```python
from build123d import *

# Parameters (mm, degrees)
F0_W     = 25
F0_H     = 300
F0_R     = 7.5
F0_R_2   = 4.25
F1_DEPTH = 50


with BuildPart() as f1:
    # F0 (on Top) → F1 (new body, symmetric)
    with BuildSketch(Plane.XY):
        Rectangle(F0_W, F0_H)
        with Locations((0, -115)):
            Circle(F0_R, mode=Mode.SUBTRACT)
        Circle(F0_R_2, mode=Mode.SUBTRACT)
        with Locations((0, 115)):
            Circle(F0_R, mode=Mode.SUBTRACT)
    extrude(amount=F1_DEPTH, both=True)


solid = f1.part
```
Read the model definition and answer for the solid it produces. Units are mm, in the model's axes. Give positions to 0.01 mm unless a question says otherwise; leave off trailing zeros. Order: outer loops, then holes, each group sorted by start corner. A loop starts at its lowest first (then second) coordinate and runs counter-clockwise, first axis right, second up.
(1) Find section D-D (y = 0). Give the vertices of the cut face in (x, z), plus the area to 3 significant figures.
(2) Find section B-B (x = 0). Give the vertices of the cut face in (y, z).
(3) Straight lines are drawn through the part: L1, parallel to Y at x = 0, z = 7; L2, parallel to Y at x = -3, z = -19.5; L3, parallel to Y at x = -6, z = 9. For each, find the intervals that lie inside material, in ascending order.
(4) For a pull along Y with two mould halves and no side action, classify faces 1 (the flat face through (0, -150, 1)), 2 (the flat face through (-6, 2, 50)), 3 (the cylindrical face through (-1.63, -122.32, -0.7)) as released by +Y, released by -Y, zero draft, split by the parting line, or undercut.
(5) Find section A-A (y = -115). Give the vertices of the cut face in (x, z).
(6) Find section C-C (z = -38.5). Give the vertices of the cut face in (x, y), plus the area to 3 significant figures.
Result sheet:
1. outline: (-12.5, -50) - (-4.25, -50) - (-4.25, 50) - (-12.5, 50) - close; (4.25, -50) - (12.5, -50) - (12.5, 50) - (4.25, 50) - close
1. area: 1,650 mm2
2. outline: (-150, -50) - (-122.5, -50) - (-122.5, 50) - (-150, 50) - close; (-107.5, -50) - (-4.25, -50) - (-4.25, 50) - (-107.5, 50) - close; (4.25, -50) - (107.5, -50) - (107.5, 50) - (4.25, 50) - close; (122.5, -50) - (150, -50) - (150, 50) - (122.5, 50) - close
3. L1: y = -150 to -122.5, -107.5 to -4.25, 4.25 to 107.5, 122.5 to 150
3. L2: y = -150 to -121.87, -108.13 to -3.01, 3.01 to 108.13, 121.87 to 150
3. L3: y = -150 to -119.5, -110.5 to 110.5, 119.5 to 150
4. face 1: released by -Y
4. face 2: zero draft
4. face 3: undercut
5. outline: (-12.5, -50) - (-7.5, -50) - (-7.5, 50) - (-12.5, 50) - close; (7.5, -50) - (12.5, -50) - (12.5, 50) - (7.5, 50) - close
6. outline: (-12.5, -150) - (12.5, -150) - (12.5, 150) - (-12.5, 150) - close; hole circle Ø15 at (0, -115); hole circle Ø15 at (0, 115); hole circle Ø8.5 at (0, 0)
6. area: 7,090 mm2
